Input: dimensioned drawing with shaded views. Units: mm. Origin: part minimum x, y, z. A direction names the side the tool comes from. Give positions to 0.01 mm unless a question says otherwise; leave off trailing zeros. Order: outer loops, then holes, each group sorted by start corner. A loop starts at its lowest first (then second) coordinate and runs counter-clockwise, first axis right, second up. Notation, with made-up numbers: M 5.5,74 L 58.5,74 A3 cw 58.5,78 Z; hole C 68,-37 d1. An arc over 180 degrees is marked long. Answer in a Markdown table with one row per item. Add a question column.
(1) Set-up query: the marked faces 1, 2, 3, 4 and 5. Return all of +Z, -Z, +X, -X, +Y, -Y with unobstructed straight access to the full face (end or side cutting, diameter ignored); none if empty.
(2) Section query D-D, the plane x = 7.75. Return loops of the section in (y, z) (1 decimal).
(3) Mould query, pull axis Z, two halves, no side actions, for the marked faces 6, 7 and 8. Classes: pulls with the +Z half, pulls with the -Z half, needs draft (parallel to the pull), parting line crosses it, or undercut.
(4) Section query B-B, the plane y = 4.5. Return loops of the section in (x, z).
(5) Section query A-A, the plane z = 29. Return loops of the section in (x, y).
(6) Section query C-C, the plane x = 13. Count the separate pieces of the cut face and the enclosed holes in it.
(7) Material intervals for line 1 along Z through (x, y) = (13, 6.5); line 2 along Z through (x, y) = (20, 0.5) (1 decimal); line 3 along Z through (x, y) = (13, 5.95), sorted ascending.
(8) Pin query (flat end, axial travel): P1, Ø1.4, axis at x = 13, y = 4, coming from the +Z side; P2, Ø2, axis at x = 9, y = 3.5, coming from the -Z side; P3, Ø6.5, axis at x = 17.5, z = 24.5, coming from the +Y side. Return the tip coordinate at first contact, or that it passes through.
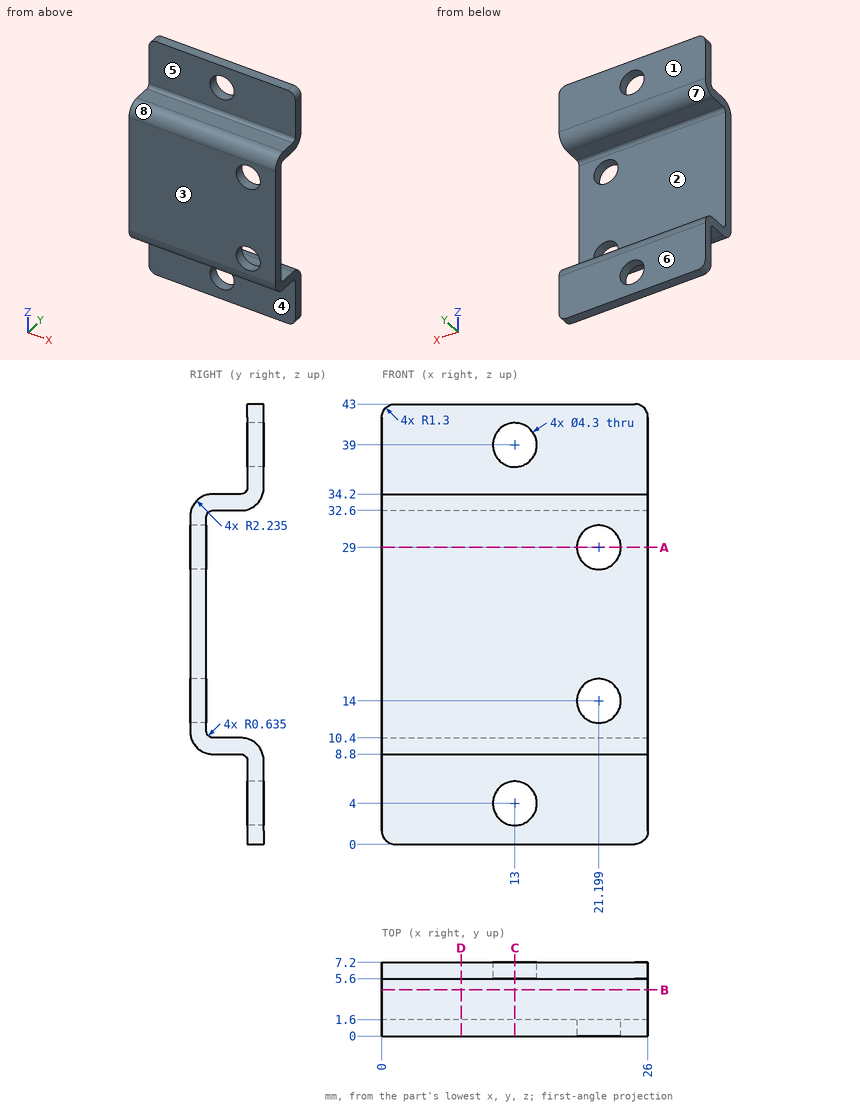
Values follow:
| question | item | result |
|---|---|---|
| 1 | face 1 | +Z, -Z, +X, -X, +Y |
| 1 | face 2 | +X, -X, +Y |
| 1 | face 3 | +Z, -Z, +X, -X, -Y |
| 1 | face 4 | -Z, +X, -X, -Y |
| 1 | face 5 | +Z, +X, -X, -Y |
| 2 | outline | M 0,11 A2.2 ccw 2.2,8.8 L 5,8.8 A0.6 cw 5.6,8.2 L 5.6,0 L 7.2,0 L 7.2,8.2 A2.2 ccw 5,10.4 L 2.2,10.4 A0.6 cw 1.6,11 L 1.6,32 A0.6 cw 2.2,32.6 L 5,32.6 A2.2 ccw 7.2,34.8 L 7.2,43 L 5.6,43 L 5.6,34.8 A0.6 cw 5,34.2 L 2.2,34.2 A2.2 ccw 0,32 Z |
| 3 | face 6 | needs draft |
| 3 | face 7 | undercut |
| 3 | face 8 | pulls with the +Z half |
| 4 | outline | M 0,8.8 L 26,8.8 L 26,10.4 L 0,10.4 Z; M 0,32.6 L 26,32.6 L 26,34.2 L 0,34.2 Z |
| 5 | outline | M 0,0 L 19.05,0 L 19.05,1.6 L 0,1.6 Z; M 23.35,0 L 26,0 L 26,1.6 L 23.35,1.6 Z |
| 6 | separate pieces | 3 |
| 6 | enclosed holes | 0 |
| 7 | line 1 | z = 0 to 1.85, 6.15 to 9.79, 33.21 to 36.85, 41.15 to 43 |
| 7 | line 2 | z = 9.6 to 12.2, 15.8 to 27.2, 30.8 to 33.4 |
| 7 | line 3 | z = 0 to 1.85, 6.15 to 10.17, 32.83 to 36.85, 41.15 to 43 |
| 8 | P1 | stops at z = 34.2 |
| 8 | P2 | stops at z = 8.8 |
| 8 | P3 | stops at y = 1.6 |
